from build123d import *

# Parameters (mm, degrees)
SALIENTE_EXTRUIR1_DEPTH = 45
CROQUIS2_R              = 3.075
CORTAR_EXTRUIR1_DEPTH   = 129.937969582
REDONDEO1_R             = 2


with BuildPart() as part:
    # Croquis1 → Saliente-Extruir1 (new body)
    with BuildSketch(Plane(origin=(0, 0, 0), x_dir=(1, 0, 0), z_dir=(0, 1, 0))):
        with BuildLine():
            Line((0, 30), (0, 50))
            Line((0, 50), (36.66060556, 50))
            Line((36.66060556, 50), (110, 15))
            Line((110, 15), (110, -15))
            Line((110, -15), (36.66060556, -50))
            Line((36.66060556, -50), (0, -50))
            Line((0, -50), (0, -30))
            ThreePointArc((0, -30), (30, 0), (0, 30))
        make_face()
    extrude(amount=SALIENTE_EXTRUIR1_DEPTH)

    # Croquis2 → Cortar-Extruir1 (cut, through all)
    with BuildSketch(Plane(origin=(110, 0, 0), x_dir=(0, 0, -1), z_dir=(1, 0, 0))):
        with Locations((0, 36.5)):
            Circle(CROQUIS2_R)
        with Locations((0, 8.5)):
            Circle(CROQUIS2_R)
    extrude(amount=-CORTAR_EXTRUIR1_DEPTH, mode=Mode.SUBTRACT)

    # Redondeo1
    redondeo1_edges = [part.edges().sort_by_distance(p)[0] for p in [
        (73.33030278, 0, 32.5),
        (73.33030278, 45, 32.5),
        (73.33030278, 45, -32.5),
        (73.33030278, 0, -32.5),
    ]]
    fillet(redondeo1_edges, radius=REDONDEO1_R)


solid = part.part
Read the model definition and answer for the solid it produces. Units are mm, in the model's axes. Round coordinates to 2 decimals unless told otherwise and drop trailing zeros. Loops run counter-clockwise (first coordinate to the right, second up) from the corner with the lowest first, then second, coordinate; pieces in that order, holes last.
Q1. Section A-A on y = 36.5 is taken. Write down the section's boundary in (x, z) (3 decimals), and give its area (3 significant figures).
Q2. Section B-B on z = 0 is taken. Write down the section's boundary in (x, y) (3 decimals).
Q3. Consider probe 1 along Y at (x, z) = (51, 0) (3 decimals); probe 2 along Z at (x, y) = (72, 36.5) (3 decimals); probe 3 along Z at (x, y) = (51, 9). Determine where each line is inside the solid, lowest interval first.
Q4. Determine the mould class of faces 1 (the face through (0, 22, 40)), 2 (the face through (72.817, 22.213, -32.745)), 3 (the face through (70.482, 5.772, -1.419)) for opening direction Z: released by +Z, released by -Z, zero draft, split by the parting line, or undercut.
Q5. Section D-D on x = 97 is taken. Give the number of separate pieces and of enclosed holes in the cut face, and give its area (3 significant figures).
Q6. Section C-C on x = 24.5 is taken. Write down the section's boundary in (y, z), and give its area (3 significant figures).
Q7. Each of these flat-tipped pins is pushed along its axis until it touches: pin 1 (8 mm diameter, centred on x = 66, z = -38.5, fed in from -Y); pin 2 (8 mm diameter, centred on y = 32.5, z = 9.5, fed in from -X); pin 3 (12 mm diameter, centred on y = 16.5, z = 16, fed in from -X). Where does it stop, or does it pass through?
Output:
1. outline: (0, -50) - (36.661, -50) - (110, -15) - (110, -3.075) - (29.842, -3.075) arc R30 cw to (0, -30) - close; (0, 30) arc R30 cw to (29.842, 3.075) - (110, 3.075) - (110, 15) - (36.661, 50) - (0, 50) - close
1. area: 6,530 mm2
2. outline: (30, 0) - (110, 0) - (110, 5.425) - (30, 5.425) - close; (30, 11.575) - (110, 11.575) - (110, 33.425) - (30, 33.425) - close; (30, 39.575) - (110, 39.575) - (110, 45) - (30, 45) - close
3. probe 1: y = 0 to 5.425, 11.575 to 33.425, 39.575 to 45
3. probe 2: z = -33.135 to -3.075, 3.075 to 33.135
3. probe 3: z = -43.16 to -3.03, 3.03 to 43.16
4. face 1: zero draft
4. face 2: released by -Z
4. face 3: undercut
5. separate pieces: 1
5. enclosed holes: 2
5. area: 1,850 mm2
6. outline: (0, -50) - (45, -50) - (45, -17.31) - (0, -17.31) - close; (0, 17.31) - (45, 17.31) - (45, 50) - (0, 50) - close
6. area: 2,940 mm2
7. pin 1: stops at y = 0.02
7. pin 2: stops at x = 26.79
7. pin 3: stops at x = 20.4
